from build123d import *

# Parameters (mm, degrees)
SKETCH_1_R          = 28
EXTRUDE_1_DEPTH     = 3
SKETCH_7_R          = 3.7
CUT_EXTRUDE_1_DEPTH = 10
SKETCH_8_R          = 3.7
CUT_EXTRUDE_2_DEPTH = 10
SKETCH_9_R          = 3.7
CUT_EXTRUDE_3_DEPTH = 10
EXTRUDE_START       = -2
SKETCH_1_3_R        = 28
EXTRUDE_3_DEPTH     = 2
SKETCH_9_2_R        = 3.7
CUT_EXTRUDE_4_DEPTH = 5
SKETCH_8_2_R        = 3.7
CUT_EXTRUDE_5_DEPTH = 5
SKETCH_7_2_R        = 3.7
CUT_EXTRUDE_6_DEPTH = 5


with BuildPart() as part:
    # Sketch 1 → Extrude 1 (new body)
    with BuildSketch(Plane(origin=(0, 0, 0), x_dir=(1, 0, 0), z_dir=(0, 1, 0))):
        with Locations(Location((0, 0, 0), (0, 0, 270))):
            Circle(SKETCH_1_R)
    extrude(amount=EXTRUDE_1_DEPTH)

    # Sketch 7 → Cut-Extrude 1 (cut)
    with BuildSketch(Plane(origin=(0, 3, 0), x_dir=(1, 0, 0), z_dir=(0, 1, 0))):
        with Locations(Location((23, 0, 0), (0, 0, 270))):
            Circle(SKETCH_7_R)
    extrude(amount=-CUT_EXTRUDE_1_DEPTH, mode=Mode.SUBTRACT)

    # Sketch 8 → Cut-Extrude 2 (cut)
    with BuildSketch(Plane(origin=(0, 3, 0), x_dir=(1, 0, 0), z_dir=(0, 1, 0))):
        with Locations(Location((-23, 0, 0), (0, 0, 270))):
            Circle(SKETCH_8_R)
    extrude(amount=-CUT_EXTRUDE_2_DEPTH, mode=Mode.SUBTRACT)

    # Sketch 9 → Cut-Extrude 3 (cut)
    with BuildSketch(Plane(origin=(0, 3, 0), x_dir=(1, 0, 0), z_dir=(0, 1, 0))):
        with Locations(Location((0, -23, 0), (0, 0, 270))):
            Circle(SKETCH_9_R)
    extrude(amount=-CUT_EXTRUDE_3_DEPTH, mode=Mode.SUBTRACT)

    # Sketch 1_3 → Extrude 3 (add)
    with BuildSketch(Plane(origin=(0, 0, 0), x_dir=(1, 0, 0), z_dir=(0, 1, 0)).offset(EXTRUDE_START)):
        with Locations(Location((0, 0, 0), (0, 0, 270))):
            Circle(SKETCH_1_3_R)
    extrude(amount=EXTRUDE_3_DEPTH)

    # Sketch 9_2 → Cut-Extrude 4 (cut)
    with BuildSketch(Plane(origin=(0, 3, 0), x_dir=(1, 0, 0), z_dir=(0, 1, 0))):
        with Locations(Location((0, -23, 0), (0, 0, 270))):
            Circle(SKETCH_9_2_R)
    extrude(amount=-CUT_EXTRUDE_4_DEPTH, mode=Mode.SUBTRACT)

    # Sketch 8_2 → Cut-Extrude 5 (cut)
    with BuildSketch(Plane(origin=(0, 3, 0), x_dir=(1, 0, 0), z_dir=(0, 1, 0))):
        with Locations(Location((-23, 0, 0), (0, 0, 270))):
            Circle(SKETCH_8_2_R)
    extrude(amount=-CUT_EXTRUDE_5_DEPTH, mode=Mode.SUBTRACT)

    # Sketch 7_2 → Cut-Extrude 6 (cut)
    with BuildSketch(Plane(origin=(0, 3, 0), x_dir=(1, 0, 0), z_dir=(0, 1, 0))):
        with Locations(Location((23, 0, 0), (0, 0, 270))):
            Circle(SKETCH_7_2_R)
    extrude(amount=-CUT_EXTRUDE_6_DEPTH, mode=Mode.SUBTRACT)


solid = part.part
Input: part model. Units: mm. Frame: model coordinates. Coordinates: 2 decimals unless noted, no trailing zeros. Loops run counter-clockwise (first coordinate to the right, second up) from the corner with the lowest first, then second, coordinate; pieces in that order, holes last.
(1) Material intervals for probe 1 along X at (y, z) = (0.8, 0); probe 2 along X at (y, z) = (1.95, 23); probe 3 along X at (y, z) = (2.35, 3), sorted ascending.
(2) Section D-D on y = -0.6. Return the cut outline in (x, z).
(3) Pull-direction query (Z, two-part tool) for faces 1 (the face through (-1.417, 0.535, 26.418)), 2 (the face through (-27.334, 0.465, -6.07)), 3 (the face through (0, 3, 0)), 4 (the face through (-26.28, 0.54, 1.71)); classes: released by +Z, released by -Z, zero draft, split by the parting line, or undercut.
(4) Section B-B on z = 0. Return the cut outline in (x, y), then the cut area to 3 significant figures.
(5) Section C-C on z = 23. Return the cut outline in (x, y).
(6) Section A-A on x = 0. Return the cut outline in (y, z).
(7) First-contact query: pin 1 Ø1.5 at (x, y) = (16, -1.5) entering from -Z; pin 2 Ø3 at (x, y) = (19, -1) entering from +Z; pin 3 Ø1 at (y, z) = (-0.5, -14.5) entering from +X; pin 4 Ø6 at (x, z) = (-23, 0) entering from -Y. Flat tips, straight axial feed; report the tip coordinate or a pass-through.
Data:
1. probe 1: x = -28 to -26.7, -19.3 to 19.3, 26.7 to 28
1. probe 2: x = -15.97 to -3.7, 3.7 to 15.97
1. probe 3: x = -27.84 to -25.17, -20.83 to 20.83, 25.17 to 27.84
2. outline: circle Ø56 at (0, 0); hole circle Ø7.4 at (-23, 0); hole circle Ø7.4 at (0, 23); hole circle Ø7.4 at (23, 0)
3. face 1: undercut
3. face 2: split by the parting line
3. face 3: zero draft
3. face 4: undercut
4. outline: (-28, -2) - (-26.7, -2) - (-26.7, 3) - (-28, 3) - close; (-19.3, -2) - (19.3, -2) - (19.3, 3) - (-19.3, 3) - close; (26.7, -2) - (28, -2) - (28, 3) - (26.7, 3) - close
4. area: 206 mm2
5. outline: (-15.97, -2) - (-3.7, -2) - (-3.7, 3) - (-15.97, 3) - close; (3.7, -2) - (15.97, -2) - (15.97, 3) - (3.7, 3) - close
6. outline: (-2, -28) - (3, -28) - (3, 19.3) - (-2, 19.3) - close; (-2, 26.7) - (3, 26.7) - (3, 28) - (-2, 28) - close
7. pin 1: stops at z = -23.48
7. pin 2: stops at z = 21.86
7. pin 3: stops at x = 24.25
7. pin 4: passes through
